from build123d import *

# Parameters (mm, degrees)
F1_R     = 2.5
F2_DEPTH = 50


with BuildPart() as f2:
    # F1 (on Right) → F2 (new body)
    with BuildSketch(Plane.YZ):
        Circle(F1_R)
    extrude(amount=F2_DEPTH)


with BuildPart() as f3_1:
    # F3: copy of F2
    add(f2.part)


solid = f3_1.part
Input: part model. Units: mm. Frame: model coordinates. Give positions to 0.01 mm unless a question says otherwise; leave off trailing zeros. Order: outer loops, then holes, each group sorted by start corner. A loop starts at its lowest first (then second) coordinate and runs counter-clockwise, first axis right, second up. Notation, with made-up numbers: M 19,76.5 L 34,76.5 A30 ccw 34,109.5 Z; hole C -24.5,54 d10. An arc over 180 degrees is marked long. Answer as a JSON object with one key per item and string values.
1. First-contact query: P1, Ø1.5, axis at x = 23.5, y = 1, coming from the +Z side; P2, Ø1.5, axis at x = 24.5, y = -2, coming from the +Z side. Flat tips, straight axial feed; report the tip coordinate or a pass-through.
Result sheet:
{"P1": "z = 2.49", "P2": "z = 2.17"}
2. Cut plane A-A, the plane x = 39. Output: boundary loops of the cut face in (y, z).
Result sheet:
{"outline": "C 0,0 d5"}
3. Cut plane C-C, the plane y = -2.05. Output: boundary loops of the cut face in (x, z).
Result sheet:
{"outline": "M 0,-1.43 L 50,-1.43 L 50,1.43 L 0,1.43 Z"}
4. Ray query, line 1 (Y direction, x = 7, z = 0.2); line 2 (Z direction, x = 8.5, y = -0.1); line 3 (Y direction, x = 41.5, z = -2.1). Return the intervals inside material, ascending. Write a range as [from, to].
Result sheet:
{"line 1": "[-2.49, 2.49]", "line 2": "[-2.5, 2.5]", "line 3": "[-1.36, 1.36]"}
5. Cut plane B-B, the plane z = -1.95. Output: boundary loops of the cut face in (x, y), and give its area (3 significant figures).
Result sheet:
{"outline": "M 0,-1.56 L 50,-1.56 L 50,1.56 L 0,1.56 Z", "area": "156 mm²"}
